from build123d import *

# Parameters (mm, degrees)
SKETCH1_R                                            = 20
BOSS_EXTRUDE1_DEPTH                                  = 6.5
CSK_FOR_M3_HEX_SOCKET_COUNTERSUNK_HEAD_S_D           = 3.4
CSK_FOR_M3_HEX_SOCKET_COUNTERSUNK_HEAD_S_CSINK_D     = 6.94
CSK_FOR_M3_HEX_SOCKET_COUNTERSUNK_HEAD_S_CSINK_ANGLE = 90
F_12_2_12_2_DIAMETER_HOLE1_D                         = 12.2
BOSS_EXTRUDE2_START                                  = -6.5
BOSS_EXTRUDE2_DEPTH                                  = 6.5
SKETCH7_W                                            = 40
SKETCH7_H                                            = 45
BOSS_EXTRUDE3_DEPTH                                  = 6
M3_CLEARANCE_HOLE2_D                                 = 3.6
CUT_EXTRUDE1_DEPTH                                   = 77.085478247
CUT_EXTRUDE1_DEPTH_BACK                              = 77.085478247
BOSS_EXTRUDE4_DEPTH                                  = 6
CHAMFER1_START                                       = -45
CHAMFER1_DEPTH                                       = 8
CHAMFER1_START_2                                     = -44
CHAMFER1_2_DEPTH                                     = 6
BOSS_EXTRUDE5_DEPTH                                  = 6
BOSS_EXTRUDE6_START                                  = -40
BOSS_EXTRUDE6_DEPTH                                  = 6


with BuildPart() as part:
    # Sketch1 → Boss-Extrude1 (new body)
    with BuildSketch(Plane.XY):
        with Locations(Location((0, 0, 0), (0, 0, 180))):
            Circle(SKETCH1_R)
    extrude(amount=BOSS_EXTRUDE1_DEPTH)

    # CSK for M3 Hex Socket Countersunk Head Screw1 (through all)
    with Locations(Plane.XY.offset(6.5)):
        with Locations((-7.75, -13.423393759), (-15.5, 0), (-7.75, 13.423393759), (7.75, 13.423393759), (15.5, 0), (7.75, -13.423393759)):
            CounterSinkHole(CSK_FOR_M3_HEX_SOCKET_COUNTERSUNK_HEAD_S_D / 2, CSK_FOR_M3_HEX_SOCKET_COUNTERSUNK_HEAD_S_CSINK_D / 2, counter_sink_angle=CSK_FOR_M3_HEX_SOCKET_COUNTERSUNK_HEAD_S_CSINK_ANGLE)

    # Ø12.2 (12.2) Diameter Hole1 (through all)
    with Locations(Plane.XY.offset(6.5)):
        with Locations((0, -7)):
            Hole(F_12_2_12_2_DIAMETER_HOLE1_D / 2)

    # Sketch6 → Boss-Extrude2 (add)
    with BuildSketch(Plane.XY.offset(6.5).offset(BOSS_EXTRUDE2_START)):
        with BuildLine():
            Line((-20, 0), (-20, -38))
            Line((-20, -38), (20, -38))
            Line((20, -38), (20, 0))
            ThreePointArc((20, 0), (0, -20), (-20, 0))
        make_face()
    extrude(amount=BOSS_EXTRUDE2_DEPTH)

    # Sketch7 → Boss-Extrude3 (add)
    with BuildSketch(Plane.XZ.offset(38)):
        with Locations((0, 22.5)):
            Rectangle(SKETCH7_W, SKETCH7_H)
    extrude(amount=BOSS_EXTRUDE3_DEPTH)

    # M3 Clearance Hole2 (through all)
    with Locations(Plane(origin=(0, -44, 0), x_dir=(-1, 0, 0), z_dir=(0, -1, 0))):
        with Locations((-17.5, -39.802814471), (17.5, -39.802814471)):
            Hole(M3_CLEARANCE_HOLE2_D / 2)

    # Sketch11 → Cut-Extrude1 (cut, two sides: drawn at the far end of the back side and taken through both)
    with BuildSketch(Plane(origin=(0, -38, 0), x_dir=(1, 0, 0), z_dir=(0, 1, 0)).offset(-CUT_EXTRUDE1_DEPTH_BACK)):
        with BuildLine():
            Line((-15.7, -37.802814471), (-15.7, -41.802814471))
            ThreePointArc((-15.7, -41.802814471), (-17.5, -43.602814471), (-19.3, -41.802814471))
            Line((-19.3, -41.802814471), (-19.3, -37.802814471))
            ThreePointArc((-19.3, -37.802814471), (-17.5, -36.002814471), (-15.7, -37.802814471))
        make_face()
        with BuildLine():
            Line((15.7, -37.802814471), (15.7, -41.802814471))
            ThreePointArc((15.7, -41.802814471), (17.5, -43.602814471), (19.3, -41.802814471))
            Line((19.3, -41.802814471), (19.3, -37.802814471))
            ThreePointArc((19.3, -37.802814471), (17.5, -36.002814471), (15.7, -37.802814471))
        make_face()
    extrude(amount=CUT_EXTRUDE1_DEPTH + CUT_EXTRUDE1_DEPTH_BACK, mode=Mode.SUBTRACT)

    # Sketch10 → Boss-Extrude4 (add)
    # profile 1 of 2: a face of its own
    with BuildSketch(Plane.XZ.offset(44)):
        with BuildLine():
            Line((-22.3, 37.802814471), (-22.3, 41.802814471))
            ThreePointArc((-22.3, 41.802814471), (-17.5, 46.602814471), (-12.7, 41.802814471))
            Line((-12.7, 41.802814471), (-12.7, 37.802814471))
            ThreePointArc((-12.7, 37.802814471), (-17.5, 33.002814471), (-22.3, 37.802814471))
        make_face()
        with BuildLine():
            Line((-19.3, 37.802814471), (-19.3, 41.802814471))
            ThreePointArc((-19.3, 41.802814471), (-17.5, 43.602814471), (-15.7, 41.802814471))
            Line((-15.7, 41.802814471), (-15.7, 37.802814471))
            ThreePointArc((-15.7, 37.802814471), (-17.5, 36.002814471), (-19.3, 37.802814471))
        make_face(mode=Mode.SUBTRACT)
    # profile 2 of 2: a face of its own
    with BuildSketch(Plane.XZ.offset(44)):
        with BuildLine():
            Line((22.3, 41.802814471), (22.3, 37.802814471))
            ThreePointArc((22.3, 37.802814471), (17.5, 33.002814471), (12.7, 37.802814471))
            Line((12.7, 37.802814471), (12.7, 41.802814471))
            ThreePointArc((12.7, 41.802814471), (17.5, 46.602814471), (22.3, 41.802814471))
        make_face()
        with BuildLine():
            Line((19.3, 41.802814471), (19.3, 37.802814471))
            ThreePointArc((19.3, 37.802814471), (17.5, 36.002814471), (15.7, 37.802814471))
            Line((15.7, 37.802814471), (15.7, 41.802814471))
            ThreePointArc((15.7, 41.802814471), (17.5, 43.602814471), (19.3, 41.802814471))
        make_face(mode=Mode.SUBTRACT)
    extrude(amount=-BOSS_EXTRUDE4_DEPTH)

    # Chamfer1: read off the stored shape, not the designer's step
    # Chamfer1 outline → Chamfer1 (cut)
    with BuildSketch(Plane(origin=(0, 0, 0), x_dir=(1, 0, 0), z_dir=(0, 1, 0)).offset(CHAMFER1_START)):
        with BuildLine():
            Line((20.05286265, -33.7379784), (21.57746495, -35.270171666))
            ThreePointArc((21.57746495, -35.270171666), (20.902530686, -34.417140989), (20.05286265, -33.7379784))
        make_face()
        with BuildLine():
            ThreePointArc((-20.05286265, -33.7379784), (-20.902530686, -34.417140989), (-21.57746495, -35.270171666))
            Line((-21.57746495, -35.270171666), (-20.05286265, -33.7379784))
        make_face()
    extrude(amount=CHAMFER1_DEPTH, mode=Mode.SUBTRACT)

    # Chamfer1 2 outline → Chamfer1 2 (add)
    with BuildSketch(Plane(origin=(0, 0, 0), x_dir=(1, 0, 0), z_dir=(0, 1, 0)).offset(CHAMFER1_START_2)):
        with BuildLine():
            ThreePointArc((20, -33.705254222), (20.026484308, -33.721530722), (20.05286265, -33.7379784))
            Line((20.05286265, -33.7379784), (20, -33.684852548))
            Line((20, -33.684852548), (20, -33.705254222))
        make_face()
        with BuildLine():
            Line((-20, -33.684852548), (-20.05286265, -33.7379784))
            ThreePointArc((-20.05286265, -33.7379784), (-20.026484308, -33.721530722), (-20, -33.705254222))
            Line((-20, -33.705254222), (-20, -33.684852548))
        make_face()
    extrude(amount=CHAMFER1_2_DEPTH)

    # Sketch12 → Boss-Extrude5 (add)
    with BuildSketch(Plane(origin=(20, 0, 0), x_dir=(0, 0, -1), z_dir=(1, 0, 0))):
        Polygon((-6.5, -30), (-14.5, -38), (-6.5, -38), align=None)
    extrude(amount=-BOSS_EXTRUDE5_DEPTH)

    # Sketch12<2> → Boss-Extrude6 (add)
    with BuildSketch(Plane(origin=(20, 0, 0), x_dir=(0, 0, -1), z_dir=(1, 0, 0)).offset(BOSS_EXTRUDE6_START)):
        Polygon((-6.5, -30), (-14.5, -38), (-6.5, -38), align=None)
    extrude(amount=BOSS_EXTRUDE6_DEPTH)


solid = part.part
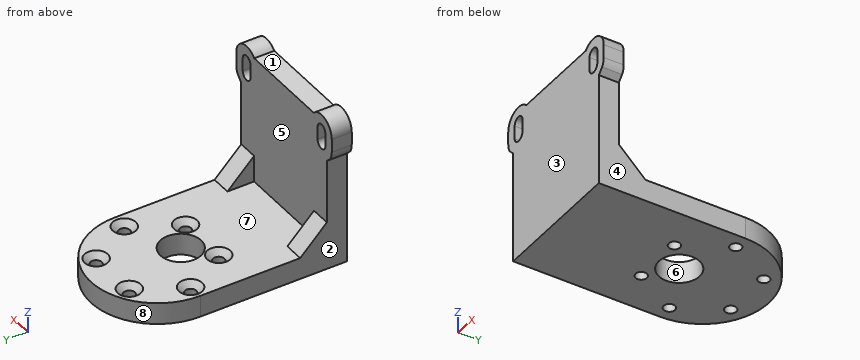
Source: CAD feature listing. Evaluate the final solid. Frame: model axes, mm. Face numbers are marked on the shaded views. A direction names the side the tool comes from. Give positions to 0.01 mm unless a question says otherwise; leave off trailing zeros. Write each loop counter-clockwise with the first axis right and the second up, starting at its lowest first coordinate (ties: lowest second). Pieces come first, ordered by that corner, then holes. Notation, with made-up numbers: (81, -35.5) -> (122, -35.5) arc R33 ccw to (122, 1.5) -> close; hole circle Ø6 at (9.5, 83.25). An arc over 180 degrees is marked (long way). Write item = value, one per line.
Q1. Mould query, pull axis Y, two halves, no side actions, for the marked faces 6, 7 and 8. Classes: +Y half, -Y half, draft (parallel to the pull), parting line (faces both ways), or undercut.
Here are the results:
face_6 = undercut
face_7 = draft
face_8 = +Y half
Q2. Reachability of the marked faces 1, 2, 3, 4 and 5 from +Z, -Z, +X, -X, +Y, -Y: full face, straight path, thin tool, end or side. Return the list, or none.
Here are the results:
face_1 = +Z, +Y, -Y
face_2 = -Z, -X, +Y, -Y
face_3 = +Z, -Z, +X, -X, -Y
face_4 = -Z, +X, +Y, -Y
face_5 = +Z, +Y
Q3. First-contact query: pin 1 (6 mm diameter, centred on x = -5.5, y = 0, fed in from +Z); pin 2 (3 mm diameter, centred on x = 7.75, y = 13.42, fed in from -Z); pin 3 (3 mm diameter, centred on x = 13.5, z = 7, fed in from +Y); pin 4 (4 mm diameter, centred on y = -33.5, z = 11.5, fed in from +X). Flat tips, straight axial feed; report the tip coordinate or a pass-through.
Here are the results:
pin_1 = 6.5
pin_2 = through
pin_3 = 15.94
pin_4 = 20
Q4. Cut plane A-A on z = 39. Return loops of the section in (x, y).
Here are the results:
outline = (-22.3, -44) -> (-19.3, -44) -> (-19.3, -38) -> (-22.3, -38) -> close; (-15.7, -44) -> (15.7, -44) -> (15.7, -38) -> (-15.7, -38) -> close; (19.3, -44) -> (22.3, -44) -> (22.3, -38) -> (19.3, -38) -> close
Q5. Cut plane C-C on x = -1. Return loops of the section in (y, z), then the cut area to 3 significant figures.
Here are the results:
outline = (-44, 0) -> (-13.02, 0) -> (-13.02, 6.5) -> (-38, 6.5) -> (-38, 45) -> (-44, 45) -> close; (-0.98, 0) -> (19.97, 0) -> (19.97, 6.5) -> (-0.98, 6.5) -> close
area = 569 mm²
Q6. Cut plane D-D on z = 4. Return loops of the section in (x, y).
Here are the results:
outline = (-20, -44) -> (20, -44) -> (20, 0) arc R20 ccw to (-20, 0) -> close; hole circle Ø3.4 at (-15.5, 0); hole circle Ø3.4 at (-7.75, -13.42); hole circle Ø3.4 at (-7.75, 13.42); hole circle Ø12.2 at (0, -7); hole circle Ø3.4 at (7.75, -13.42); hole circle Ø3.4 at (7.75, 13.42); hole circle Ø3.4 at (15.5, 0)
Q7. Line query: line 1 (Y direction, x = 0, z = 4); line 2 (Y direction, x = 7.75, z = 1); line 3 (Y direction, x = -4, z = 34.5). Output: solid intervals per line, ascending. Write a range as from..to.
Here are the results:
line_1 = -44..-13.1, -0.9..20
line_2 = -44..-15.12, -11.72..11.72, 15.12..18.44
line_3 = -44..-38
Q8. Cut plane B-B on x = -7.75. Return loops of the section in (y, z), then the cut area to 3 significant figures.
Here are the results:
outline = (-44, 0) -> (-15.12, 0) -> (-15.12, 4.73) -> (-16.89, 6.5) -> (-38, 6.5) -> (-38, 45) -> (-44, 45) -> close; (-11.72, 0) -> (11.72, 0) -> (11.72, 4.73) -> (9.95, 6.5) -> (-9.95, 6.5) -> (-11.72, 4.73) -> close; (15.12, 0) -> (18.44, 0) -> (18.44, 6.5) -> (16.89, 6.5) -> (15.12, 4.73) -> close
area = 586 mm²
